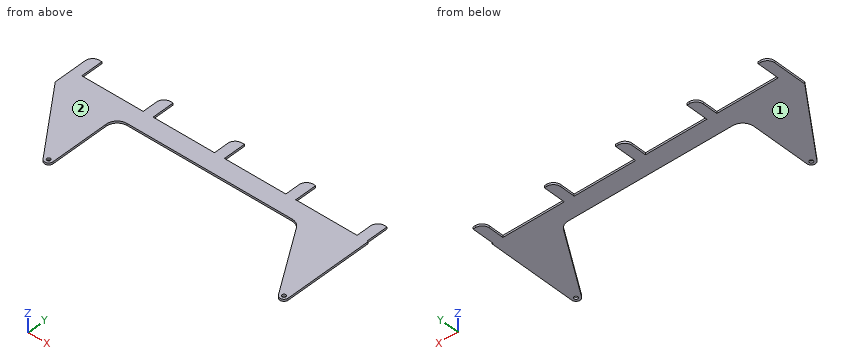
```python
from build123d import *

# Parameters (mm, degrees)
SKETCH1_R           = 5
BOSS_EXTRUDE1_DEPTH = 2.75
FILLET1_R           = 20


with BuildPart() as part:
    # Sketch1 → Boss-Extrude1 (new body, symmetric)
    with BuildSketch(Plane.XY):
        with BuildLine():
            Line((-402.92, 0), (-402.92, 60))
            Line((-402.92, 60), (-375.92, 60))
            Line((-375.92, 60), (-375.92, 0))
            Line((-375.92, 0), (-208.92, 0))
            Line((-208.92, 0), (-208.92, 60))
            Line((-208.92, 60), (-181.92, 60))
            Line((-181.92, 60), (-181.92, 0))
            Line((-181.92, 0), (-14.92, 0))
            Line((-14.92, 0), (-14.92, 60))
            Line((-14.92, 60), (12.08, 60))
            Line((12.08, 60), (12.08, 0))
            Line((12.08, 0), (179.08, 0))
            Line((179.08, 0), (179.08, 60))
            Line((179.08, 60), (206.08, 60))
            Line((206.08, 60), (206.08, 0))
            Line((206.08, 0), (373.08, 0))
            Line((373.08, 0), (373.08, 60))
            Line((373.08, 60), (400.08, 60))
            Line((400.08, 60), (400.08, 0))
            Line((400.08, 0), (402.92, 0))
            Line((402.92, 0), (402.92, -240))
            ThreePointArc((402.92, -240), (394.630398166, -251.042796005), (381.71246198, -246.165525573))
            Line((381.71246198, -246.165525573), (265.960766405, -63.916020245))
            ThreePointArc((265.960766405, -63.916020245), (255.084601896, -53.708181951), (240.636754178, -50))
            Line((240.636754178, -50), (-207.242294627, -50))
            ThreePointArc((-207.242294627, -50), (-228.455498062, -58.786796564), (-237.242294627, -80))
            Line((-237.242294627, -80), (-237.242294627, -240))
            ThreePointArc((-237.242294627, -240), (-245.153860516, -250.925801601), (-258.002840824, -246.81852507))
            Line((-258.002840824, -246.81852507), (-402.92, -50))
            Line((-402.92, -50), (-402.92, 0))
        make_face()
        with Locations((-248.742294627, -240)):
            Circle(SKETCH1_R, mode=Mode.SUBTRACT)
        with Locations((391.42, -240)):
            Circle(SKETCH1_R, mode=Mode.SUBTRACT)
    extrude(amount=BOSS_EXTRUDE1_DEPTH, both=True)

    # Fillet1
    fillet1_edges = [part.edges().sort_by_distance(p)[0] for p in [
        (-402.92, 60, 0),
        (-208.92, 60, 0),
        (-14.92, 60, 0),
        (179.08, 60, 0),
        (373.08, 60, 0),
    ]]
    fillet(fillet1_edges, radius=FILLET1_R)


solid = part.part
```
Can you work these out from the model? Positions are in its coordinate system, mm. Face numbers are marked on the shaded views. Round coordinates to 2 decimals unless told otherwise and drop trailing zeros. Loops run counter-clockwise (first coordinate to the right, second up) from the corner with the lowest first, then second, coordinate; pieces in that order, holes last. Notation, with made-up numbers: (-36, 67) -> (-16, 67) arc R20 cw to (-16, 77) -> close; hole circle Ø8 at (-31, 22.25). An arc over 180 degrees is marked (long way). One line per item, written item: value. Start each with the question number.
1. For pin 1 (8 mm diameter, centred on x = -248.74, y = -240, fed in from -Z); pin 2 (2 mm diameter, centred on x = -138, z = -2, fed in from +Y); pin 3 (3 mm diameter, centred on y = 26, z = 0.5, fed in from +X); pin 4 (3 mm diameter, centred on x = 127.5, z = 0.5, fed in from -Y), each with a flat end and sliding along its axis, tell me the tip position at first contact or that it passes through.
2. If I drill on probe 1 along X at (y, z) = (10, 1.5); probe 2 along Y at (x, z) = (391.42, 1.4); probe 3 along X at (y, z) = (43.5, 1.65), over which ranges is the centre line in solid material (lowest first)?
3. If we section it at C-C, the plane x = 254: Write out the boundary of the cut face in (y, z).
4. If we mould it in two halves opening along Z, with no side actions, what happens to the marked faces 1 and 2? For each: pulls with the +Z half, pulls with the -Z half, needs draft (parallel to the pull), parting line crosses it, or undercut.
5. If we section it at B-B, the plane z = -1.25: Give the number of separate pieces and of enclosed holes in the cut face, then the cut area to 3 significant figures.
6. If we section it at A-A, the plane x = 50: Write out the boundary of the cut face in (y, z).
Calculated:
1. pin 1: passes through
1. pin 2: stops at y = 0
1. pin 3: stops at x = 400.08
1. pin 4: stops at y = -50
2. probe 1: x = -402.92 to -375.92, -208.92 to -181.92, -14.92 to 12.08, 179.08 to 206.08, 373.08 to 400.08
2. probe 2: y = -251.5 to -245, -235 to 59.93
2. probe 3: x = -402.61 to -375.92, -208.61 to -181.92, -14.61 to 12.08, 179.39 to 206.08, 373.39 to 400.08
3. outline: (-53.14, -2.75) -> (0, -2.75) -> (0, 2.75) -> (-53.14, 2.75) -> close
4. face 1: pulls with the -Z half
4. face 2: pulls with the +Z half
5. separate pieces: 1
5. enclosed holes: 2
5. area: 82,900 mm²
6. outline: (-50, -2.75) -> (0, -2.75) -> (0, 2.75) -> (-50, 2.75) -> close
